Could you check a few things on this model? Use its own coordinates, in mm. Face numbers are marked on the shaded views. A direction names the side the tool comes from. Coordinates: 2 decimals unless noted, no trailing zeros. Loops run counter-clockwise (first coordinate to the right, second up) from the corner with the lowest first, then second, coordinate; pieces in that order, holes last.
1) Imagine slicing it at D-D on x = 8.5. Please give me the cut outline in (y, z).
2) Imagine slicing it at B-B on y = 3.75. Please give me the cut outline in (x, z).
3) Will these pins go through, and if not, where does the flat tip stop? P1, Ø1, axis at x = -13.5, y = -1.5, coming from the +Z side; P2, Ø1, axis at y = -1.5, z = -5, coming from the +X side; P3, Ø3, axis at y = 3, z = -3, coming from the -X side; P4, Ø8, axis at x = 9.5, z = -10.5, coming from the -Y side.
4) If I drill on line 1 along X through (y, z) = (4.75, -13.5); line 2 along Y through (x, z) = (-15, 7); line 3 along X through (y, z) = (0.5, 22), over which ranges is the centre line in solid material (lowest first)?
5) Imagine slicing it at A-A on z = 2. Please give me the cut outline in (x, y).
6) Imagine slicing it at C-C on y = 1. Please give me the cut outline in (x, z).
7) For the marked faces 1, 2, 3 and 4, which set-ups out of +Z, -Z, +X, -X, +Y, -Y let a thin tool reach every point of the face, with its end or its side?
8) Thinking about a two-plate mould opening in X: for the marked faces 5, 6 and 7, which applies, released by +X, released by -X, zero draft, split by the parting line, or undercut?
```python
from build123d import *

# Parameters (mm, degrees)
F1_DEPTH    = 2.921
F3_DEPTH    = 5.842
F4_T1_DEPTH = 5.842
F5_T1_DEPTH = 90.842
F7_DEPTH    = 1.3335
F9_DEPTH    = 1.3335


# Not quite as in the source:
# - a fillet or chamfer that OpenCascade refuses, or shapes differently, is made with other operations: its cross-section is extruded or revolved along the edge and cut away or added


with BuildPart() as f1:
    # F0 (on Front) → F1 (new body, symmetric)
    with BuildSketch(Plane.XZ):
        Polygon((-14.351, -21.6027), (-14.351, 21.6027), (14.351, 21.6027), (14.351, -21.6027), (15.6845, -21.6027), (15.6845, 24.1027), (-15.6845, 24.1027), (-15.6845, -21.6027), align=None)
    extrude(amount=F1_DEPTH, both=True)

    # F2 (on face) → F3 (join, through all)
    with BuildSketch(Plane.XZ.offset(2.921)):
        Polygon((-14.351, -23.6027), (-14.351, -21.6027), (-15.6845, -21.6027), (-19.351, -21.6027), (-19.351, -23.6027), align=None)
        Polygon((15.6845, -21.6027), (14.351, -21.6027), (14.351, -23.6027), (19.351, -23.6027), (19.351, -21.6027), align=None)
    extrude(amount=-F3_DEPTH)

    # F4: fillet of radius 15 on 2 edges, made by hand

    # F4_s2 → F4_t1 (join)
    with BuildSketch(Plane.XZ.offset(-2.921)):
        with BuildLine():
            ThreePointArc((-14.351, 6.6027), (-9.9576017178, 17.2093017178), (0.649, 21.6027))
            Line((0.649, 21.6027), (-14.351, 21.6027))
            Line((-14.351, 21.6027), (-14.351, 6.6027))
        make_face()
        with BuildLine():
            ThreePointArc((14.351, 6.6027), (9.9576017178, 17.2093017178), (-0.649, 21.6027))
            Line((-0.649, 21.6027), (14.351, 21.6027))
            Line((14.351, 21.6027), (14.351, 6.6027))
        make_face()
    extrude(amount=F4_T1_DEPTH)

    # F5: fillet of radius 17 on 2 edges, made by hand

    # F5_s2 → F5_t1 (cut)
    with BuildSketch(Plane.XZ.offset(-45.421)):
        with BuildLine():
            ThreePointArc((1.3155, 24.1027), (-10.7053152802, 19.1235152802), (-15.6845, 7.1027))
            Line((-15.6845, 7.1027), (-15.6845, 24.1027))
            Line((-15.6845, 24.1027), (1.3155, 24.1027))
        make_face()
        with BuildLine():
            ThreePointArc((15.6845, 7.1027), (10.7053152802, 19.1235152802), (-1.3155, 24.1027))
            Line((-1.3155, 24.1027), (15.6845, 24.1027))
            Line((15.6845, 24.1027), (15.6845, 7.1027))
        make_face()
    extrude(amount=F5_T1_DEPTH, mode=Mode.SUBTRACT)

    # F6 (on face) → F7 (join, through all)
    with BuildSketch(Plane(origin=(-15.6845, 0, 0), x_dir=(0, -1, 0), z_dir=(-1, 0, 0))):
        Polygon((-2.921, -21.6027), (-2.921, 7.1027), (-7.239, -21.6027), align=None)
    extrude(amount=-F7_DEPTH)

    # F8 (on face) → F9 (join, through all)
    with BuildSketch(Plane.YZ.offset(15.6845)):
        Polygon((2.921, 6.6027), (2.921, -21.6027), (7.239, -21.6027), (2.921, 7.1027), align=None)
    extrude(amount=-F9_DEPTH)


solid = f1.part
```
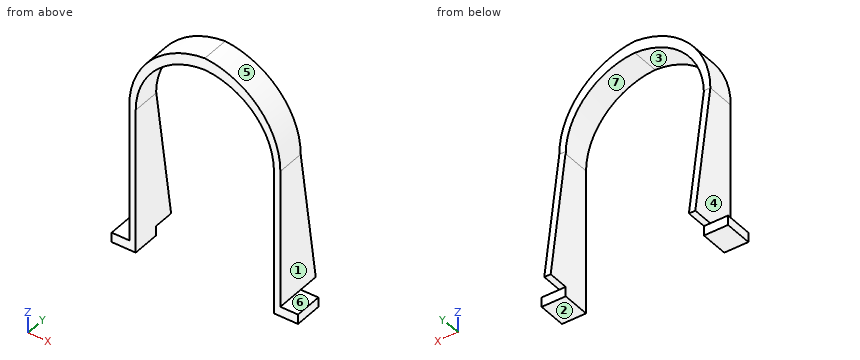
Filled in:
1. outline: (-2.92, 18.49) - (2.92, 18.49) - (2.92, 20.98) - (-2.92, 20.98) - close
2. outline: (-15.68, -21.6) - (-14.35, -21.6) - (-14.35, 1.59) - (-15.68, 1.59) - close; (14.35, -21.6) - (15.68, -21.6) - (15.68, 1.59) - (14.35, 1.59) - close
3. P1: stops at z = 16.27
3. P2: stops at x = 15.68
3. P3: stops at x = -15.68
3. P4: passes through
4. line 1: x = -15.68 to -14.35, 14.35 to 15.68
4. line 2: y = -2.92 to 2.94
4. line 3: x = -6.87 to 6.87
5. outline: (-15.68, -2.92) - (-14.35, -2.92) - (-14.35, 3.69) - (-15.68, 3.69) - close; (14.35, -2.92) - (15.68, -2.92) - (15.68, 3.69) - (14.35, 3.69) - close
6. outline: (-19.35, -23.6) - (-14.35, -23.6) - (-14.35, 6.6) arc R15 cw to (0, 21.59) arc R15 cw to (14.35, 6.6) - (14.35, -23.6) - (19.35, -23.6) - (19.35, -21.6) - (15.68, -21.6) - (15.68, 7.1) arc R17 ccw to (0, 24.05) arc R17 ccw to (-15.68, 7.1) - (-15.68, -21.6) - (-19.35, -21.6) - close
7. face 1: +Z, +X, +Y, -Y
7. face 2: -Z, +X, -X, +Y, -Y
7. face 3: -Z, +Y, -Y
7. face 4: +Z, -X, +Y, -Y
8. face 5: released by +X
8. face 6: zero draft
8. face 7: undercut
